Build history of the part. All positions in model axes, mm. A direction names the side the tool comes from. Coordinates: 2 decimals unless noted, no trailing zeros. Order: outer loops, then holes, each group sorted by start corner. A loop starts at its lowest first (then second) coordinate and runs counter-clockwise, first axis right, second up. Notation, with made-up numbers: M 68.25,3.25 L 105.25,3.25 A36 cw 105.25,38.25 Z; hole C 59.25,7 d5. An arc over 180 degrees is marked long. Use a Markdown table: item, result. Add a question column.
from build123d import *

# Parameters (mm, degrees)
SKETCH1_W           = 600
SKETCH1_H           = 250
BOSS_EXTRUDE1_DEPTH = 130
SKETCH2_W           = 590
SKETCH2_H           = 240
CUT_EXTRUDE1_DEPTH  = 120
SKETCH3_W           = 590
SKETCH3_H           = 10
BOSS_EXTRUDE2_DEPTH = 20
SKETCH4_W           = 30
SKETCH4_H           = 20
SKETCH4_H_2         = 20.05334452
BOSS_EXTRUDE3_DEPTH = 200
SKETCH5_R           = 12.7
BOSS_EXTRUDE4_DEPTH = 60


with BuildPart() as part:
    # Sketch1 → Boss-Extrude1 (new body)
    with BuildSketch(Plane(origin=(0, 0, 0), x_dir=(1, 0, 0), z_dir=(0, 1, 0))):
        Rectangle(SKETCH1_W, SKETCH1_H)
    extrude(amount=BOSS_EXTRUDE1_DEPTH)

    # Sketch2 → Cut-Extrude1 (cut)
    with BuildSketch(Plane(origin=(0, 130, 0), x_dir=(1, 0, 0), z_dir=(0, 1, 0))):
        Rectangle(SKETCH2_W, SKETCH2_H)
    extrude(amount=-CUT_EXTRUDE1_DEPTH, mode=Mode.SUBTRACT)

    # Sketch3 → Boss-Extrude2 (add)
    with BuildSketch(Plane(origin=(0, 10, 0), x_dir=(1, 0, 0), z_dir=(0, 1, 0))):
        with Locations((0, -115)):
            Rectangle(SKETCH3_W, SKETCH3_H)
        with Locations((0, -55)):
            Rectangle(SKETCH3_W, SKETCH3_H)
        with Locations((0, 55)):
            Rectangle(SKETCH3_W, SKETCH3_H)
        with Locations((0, 115)):
            Rectangle(SKETCH3_W, SKETCH3_H)
    extrude(amount=BOSS_EXTRUDE2_DEPTH)

    # Sketch4 → Boss-Extrude3 (add)
    with BuildSketch(Plane.ZY.offset(300)):
        with Locations((-95, 10)):
            Rectangle(SKETCH4_W, SKETCH4_H)
        with Locations((95, 10.02667226)):
            Rectangle(SKETCH4_W, SKETCH4_H_2)
    extrude(amount=BOSS_EXTRUDE3_DEPTH)

    # Sketch5 → Boss-Extrude4 (add)
    with BuildSketch(Plane(origin=(0, 20, 0), x_dir=(1, 0, 0), z_dir=(0, 1, 0))):
        with Locations(Location((-485, -95, 0), (0, 0, 90))):
            Circle(SKETCH5_R)
        with Locations(Location((-485, 95, 0), (0, 0, 270))):
            Circle(SKETCH5_R)
    extrude(amount=BOSS_EXTRUDE4_DEPTH)


solid = part.part
(1) Which spindle directions (+Z, -Z, +X, -X, +Y, -Y) get a long thin tool onto all of the face, cutting with end or side? Do faces 5 (the flat face through (-399, 10, -80)), 6 (the flat face through (-4, 20, 50)), 7 (the flat face through (-485, 80, -95)). Say none if no direction does.
(2) Slice it at A-A on y = 55. Give the cut face in (x, z), and give its area (3 significant figures).
(3) Slice it at B-B on x = -485. Give the cut face in (y, z), and give its area (3 significant figures).
(4) Mould opens along X. For faces 1 (the flat face through (300, 64, 2)), 2 (the flat face through (-485, 80, 95)), 3 (the flat face through (-500, 10, 95)), 4 (the flat face through (-399, 20, -95)) say: released by +X, released by -X, zero draft, split by the parting line, or undercut.
(5) Slice it at C-C on x = 233. Give the cut face in (y, z).
(6) Drop flat-ended pins along their axis: P1, Ø3, axis at x = 14, z = -54.5, coming from the +Y side; P2, Ø16, axis at x = -405.5, y = 14.5, coming from the +Z side; P3, Ø24, axis at x = -385, z = 96.5, coming from the +Y side. Give the stop position or say it passes through.
(7) Slice it at D-D on z = -95. Give the cut face in (x, y).
(8) Drill centre lines: line 1 along Z through (x, y) = (2, 25); line 2 along X through (y, z) = (38, -93); line 3 along X through (y, z) = (35, 28.5). Where is each one in solid material? Low to high. Write a range as from..to.
Solutions:
| question | item | result |
|---|---|---|
| 1 | face 5 | -X, +Y, -Y |
| 1 | face 6 | +Y |
| 1 | face 7 | +Z, -Z, -X, +Y |
| 2 | outline | C -485,-95 d25.4; C -485,95 d25.4; M -300,-125 L 300,-125 L 300,125 L -300,125 Z; hole M -295,-120 L 295,-120 L 295,120 L -295,120 Z |
| 2 | area | 9,410 mm² |
| 3 | outline | M 0,-110 L 20,-110 L 20,-107.7 L 80,-107.7 L 80,-82.3 L 20,-82.3 L 20,-80 L 0,-80 Z; M 0,80 L 20.05,80 L 20.05,82.3 L 80,82.3 L 80,107.7 L 20.05,107.7 L 20.05,110 L 0,110 Z |
| 3 | area | 4,250 mm² |
| 4 | face 1 | released by +X |
| 4 | face 2 | zero draft |
| 4 | face 3 | released by -X |
| 4 | face 4 | undercut |
| 5 | outline | M 0,-125 L 130,-125 L 130,-120 L 30,-120 L 30,-110 L 10,-110 L 10,-60 L 30,-60 L 30,-50 L 10,-50 L 10,50 L 30,50 L 30,60 L 10,60 L 10,110 L 30,110 L 30,120 L 130,120 L 130,125 L 0,125 Z |
| 6 | P1 | y = 30 |
| 6 | P2 | z = 110 |
| 6 | P3 | y = 20.05 |
| 7 | outline | M -500,0 L 300,0 L 300,130 L 295,130 L 295,10 L -295,10 L -295,130 L -300,130 L -300,20 L -472.3,20 L -472.3,80 L -497.7,80 L -497.7,20 L -500,20 Z |
| 8 | line 1 | -125..-110, -60..-50, 50..60, 110..125 |
| 8 | line 2 | -497.54..-472.46, -300..-295, 295..300 |
| 8 | line 3 | -300..-295, 295..300 |
